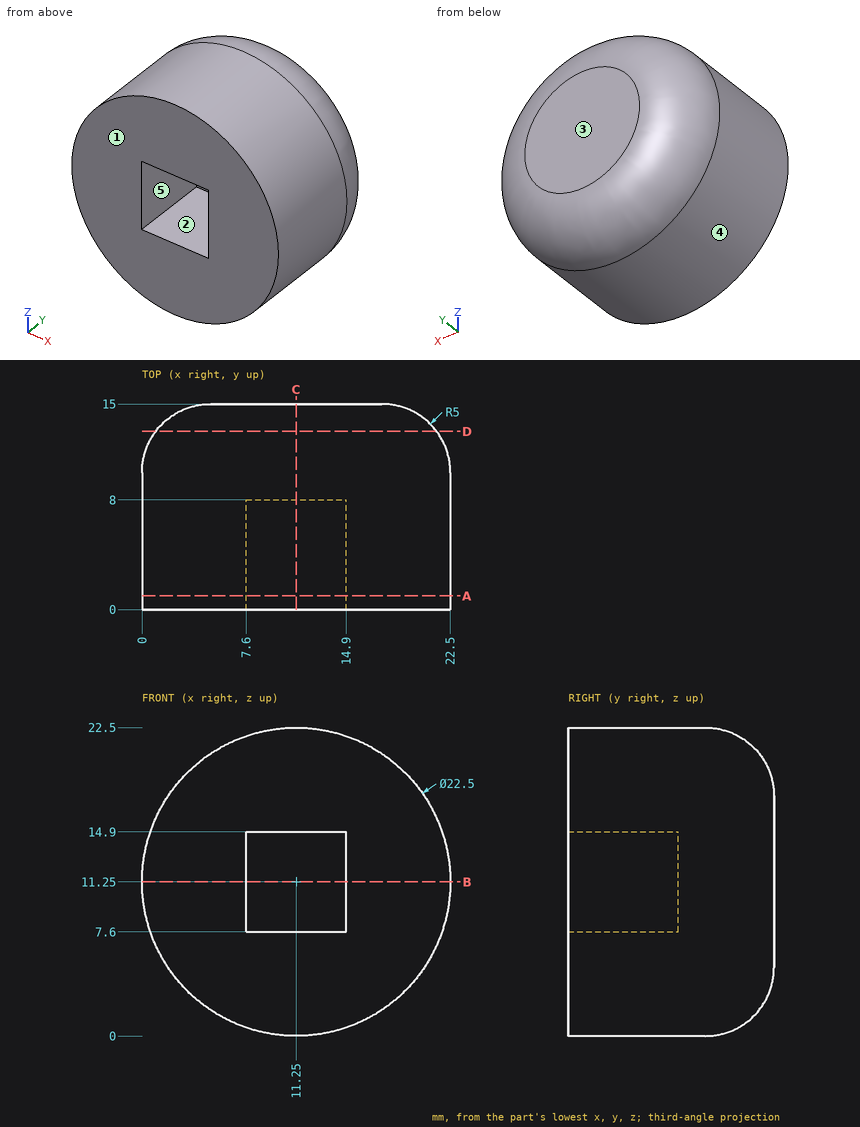
Verification items for this drawing (mm, ordinates from the low corner). A direction names the side the tool comes from. Give positions to 0.01 mm unless a question says otherwise; leave off trailing zeros. Write each loop counter-clockwise with the first axis right and the second up, starting at its lowest first coordinate (ties: lowest second). Pieces come first, ordered by that corner, then holes.
1) Cross-section at A-A (y = 1). Record the boundary of the cut face in (x, z), plus the area to 3 significant figures.
Values follow:
outline: circle Ø22.5 at (11.25, 11.25); hole (7.6, 7.6) - (14.9, 7.6) - (14.9, 14.9) - (7.6, 14.9) - close
area: 344 mm2
2) Cross-section at D-D (y = 13). Record the boundary of the cut face in (x, z), plus the area to 3 significant figures.
Values follow:
outline: circle Ø20.5 at (11.25, 11.25)
area: 330 mm2
3) Release check for a two-part mould opening along X. For the marked faces 3, 4 and 5 record: released by +X, released by -X, zero draft, split by the parting line, or undercut.
Values follow:
face 3: zero draft
face 4: split by the parting line
face 5: undercut
4) Thickness scan on line 1 (Y direction, x = 11.5, z = 9.75); line 2 (Z direction, x = 9.25, y = 7.5); line 3 (Z direction, x = 11, y = 8.5). Record the ranges inside material, lowest first.
Values follow:
line 1: y = 8 to 15
line 2: z = 0.18 to 7.6, 14.9 to 22.32
line 3: z = 0 to 22.5
5) Go/stop test with flat-tipped pins: pin 1 Ø2 at (x, y) = (13.5, 2.5) entering from -Z; pin 2 Ø2 at (x, y) = (9.5, 2) entering from +Z (3 decimals); pin 3 Ø6 at (x, y) = (19.5, 7.5) entering from +Z. Record where each tip stops, or that it passes through.
Values follow:
pin 1: stops at z = 0.07
pin 2: stops at z = 22.475
pin 3: stops at z = 21.2
6) Cross-section at C-C (x = 11.25). Record the boundary of the cut face in (y, z), plus the area to 3 significant figures.
Values follow:
outline: (0, 0) - (10, 0) arc R5 ccw to (15, 5) - (15, 17.5) arc R5 ccw to (10, 22.5) - (0, 22.5) - (0, 14.9) - (8, 14.9) - (8, 7.6) - (0, 7.6) - close
area: 268 mm2
7) Cross-section at B-B (z = 11.25). Record the boundary of the cut face in (x, y).
Values follow:
outline: (0, 0) - (7.6, 0) - (7.6, 8) - (14.9, 8) - (14.9, 0) - (22.5, 0) - (22.5, 10) arc R5 ccw to (17.5, 15) - (5, 15) arc R5 ccw to (0, 10) - close
8) Set-up check for the marked faces 1 and 2: record each of +Z, -Z, +X, -X, +Y, -Y from which the full face is reachable in a straight line by a thin tool's end or side.
Values follow:
face 1: +Z, -Z, +X, -X, -Y
face 2: -Y
